Read the model definition and answer for the solid it produces. Units are mm, in the model's axes. A direction names the side the tool comes from. Coordinates: 2 decimals unless noted, no trailing zeros. Loops run counter-clockwise (first coordinate to the right, second up) from the corner with the lowest first, then second, coordinate; pieces in that order, holes last. Notation, with made-up numbers: (89.25, 65.5) -> (148.25, 65.5) arc R16 ccw to (148.25, 69.5) -> close; hole circle Ø1 at (-6.75, 74.5). An arc over 180 degrees is marked (long way). Answer in a Markdown table with one row per item.
```python
from build123d import *

# Parameters (mm, degrees)
SKETCH_1_W          = 26.8
SKETCH_1_H          = 26.8
EXTRUDE_1_DEPTH     = 3.2
SKETCH_2_W          = 26.8
SKETCH_2_H          = 26.8
SKETCH_2_W_2        = 24.7
SKETCH_2_H_2        = 16.6
CUT_EXTRUDE_1_DEPTH = 1.5
SKETCH_3_W          = 10.4
SKETCH_3_H          = 2.6
EXTRUDE_2_DEPTH     = 17.5
SKETCH_4_W          = 23
SKETCH_4_H          = 6
EXTRUDE_3_DEPTH     = 1.5
SKETCH_5_R          = 0.98
CUT_EXTRUDE_2_DEPTH = 10


with BuildPart() as part:
    # 草图1 → 凸台-拉伸1 (new body)
    with BuildSketch(Plane(origin=(0, 0, 0), x_dir=(0, 0, -1), z_dir=(1, 0, 0))):
        Rectangle(SKETCH_1_W, SKETCH_1_H)
    extrude(amount=EXTRUDE_1_DEPTH)

    # 草图2 → 切除-拉伸1 (cut)
    with BuildSketch(Plane(origin=(3.2, 0, 0), x_dir=(0, 0, -1), z_dir=(1, 0, 0))):
        Rectangle(SKETCH_2_W, SKETCH_2_H)
        Rectangle(SKETCH_2_W_2, SKETCH_2_H_2, mode=Mode.SUBTRACT)
    extrude(amount=-CUT_EXTRUDE_1_DEPTH, mode=Mode.SUBTRACT)

    # 草图3 → 凸台-拉伸2 (add)
    with BuildSketch(Plane.ZY):
        with Locations((0, 11.6)):
            Rectangle(SKETCH_3_W, SKETCH_3_H)
    extrude(amount=EXTRUDE_2_DEPTH)

    # 草图4 → 凸台-拉伸3 (add)
    with BuildSketch(Plane.ZY):
        with Locations((0, 0.6)):
            Rectangle(SKETCH_4_W, SKETCH_4_H)
    extrude(amount=EXTRUDE_3_DEPTH)

    # 草图5 → 切除-拉伸2 (cut)
    with BuildSketch(Plane(origin=(1.7, 0, 0), x_dir=(0, 0, -1), z_dir=(1, 0, 0))):
        with Locations((-10.5, 11.1)):
            Circle(SKETCH_5_R)
        with Locations((10.5, 11.1)):
            Circle(SKETCH_5_R)
        with Locations((10.5, -11.1)):
            Circle(SKETCH_5_R)
        with Locations((-10.5, -11.1)):
            Circle(SKETCH_5_R)
    extrude(amount=-CUT_EXTRUDE_2_DEPTH, mode=Mode.SUBTRACT)


solid = part.part
```
1. The mould has two halves that part along Z. Classify faces 6 (the cylindrical face through (0.862, 11.394, -11.435)), 7 (the flat face through (-9, 12, -5.2)), 8 (the flat face through (1, -13.4, 0)): pulls with the +Z half, pulls with the -Z half, needs draft (parallel to the pull), parting line crosses it, or undercut.
A:
| item | result |
|---|---|
| face 6 | undercut |
| face 7 | pulls with the -Z half |
| face 8 | needs draft |
2. A tool of negligible diameter and unlimited length cuts with its end or side. For faces 1 (the flat face through (-9, 12.9, 0)), 2 (the flat face through (-1, -2.4, 0)), 3 (the flat face through (2, 8.3, 0)), 4 (the flat face through (2, 0, -12.35)), 5 (the flat face through (2, -8.3, 0)), from which of +Z, -Z, +X, -X, +Y, -Y can it reach the whole face along a straight path? Write none if from no direction.
A:
| item | result |
|---|---|
| face 1 | +Z, -Z, -X, +Y |
| face 2 | +Z, -Z, -X, -Y |
| face 3 | +Z, -Z, +X, +Y |
| face 4 | -Z, +X, +Y, -Y |
| face 5 | +Z, -Z, +X, -Y |
3. A cutting plane is placed at A-A on y = -11.1. Give the vertices of the cut face in (x, z), and give its area (3 significant figures).
A:
| item | result |
|---|---|
| outline | (0, -13.4) -> (1.7, -13.4) -> (1.7, -11.48) -> (0, -11.48) -> close; (0, -9.52) -> (1.7, -9.52) -> (1.7, 9.52) -> (0, 9.52) -> close; (0, 11.48) -> (1.7, 11.48) -> (1.7, 13.4) -> (0, 13.4) -> close |
| area | 38.9 mm2 |
4. Given pin 1 Ø0.8 at (x, z) = (2.5, -0.5) entering from -Y; pin 2 Ø4 at (y, z) = (-6, -7) entering from -X; pin 3 Ø5 at (x, z) = (-12, 0) entering from +Y, each flat-ended and moving along its own axis, determine where each tip first touches the part or whether it passes through.
A:
| item | result |
|---|---|
| pin 1 | stops at y = -8.3 |
| pin 2 | stops at x = 0 |
| pin 3 | stops at y = 12.9 |
5. A cutting plane is placed at C-C on z = -10.5. Give the vertices of the cut face in (x, y).
A:
| item | result |
|---|---|
| outline | (-1.5, -2.4) -> (0, -2.4) -> (0, -10.12) -> (1.7, -10.12) -> (1.7, -8.3) -> (3.2, -8.3) -> (3.2, 8.3) -> (1.7, 8.3) -> (1.7, 10.12) -> (0, 10.12) -> (0, 3.6) -> (-1.5, 3.6) -> close; (0, -13.4) -> (1.7, -13.4) -> (1.7, -12.08) -> (0, -12.08) -> close; (0, 12.08) -> (1.7, 12.08) -> (1.7, 13.4) -> (0, 13.4) -> close |
6. Find the intervals of material crossed by probe 1 along Y at (x, z) = (1, -10.5); probe 2 along X at (y, z) = (9.5, 7); probe 3 along X at (y, z) = (6, -7.75), in increasing order.
A:
| item | result |
|---|---|
| probe 1 | y = -13.4 to -12.08, -10.12 to 10.12, 12.08 to 13.4 |
| probe 2 | x = 0 to 1.7 |
| probe 3 | x = 0 to 3.2 |
7. A cutting plane is placed at D-D on y = -4.75. Give the vertices of the cut face in (x, z), and give its area (3 significant figures).
A:
| item | result |
|---|---|
| outline | (0, -13.4) -> (1.7, -13.4) -> (1.7, -12.35) -> (3.2, -12.35) -> (3.2, 12.35) -> (1.7, 12.35) -> (1.7, 13.4) -> (0, 13.4) -> close |
| area | 82.6 mm2 |
8. A cutting plane is placed at B-B on z = 4.25. Give the vertices of the cut face in (x, y), and give its area (3 significant figures).
A:
| item | result |
|---|---|
| outline | (-17.5, 10.3) -> (0, 10.3) -> (0, 3.6) -> (-1.5, 3.6) -> (-1.5, -2.4) -> (0, -2.4) -> (0, -13.4) -> (1.7, -13.4) -> (1.7, -8.3) -> (3.2, -8.3) -> (3.2, 8.3) -> (1.7, 8.3) -> (1.7, 13.4) -> (0, 13.4) -> (0, 12.9) -> (-17.5, 12.9) -> close |
| area | 125 mm2 |
